Geometry check sheet. Reference: the model listing, model coordinates, mm. A direction names the side the tool comes from. Coordinates: 2 decimals unless noted, no trailing zeros. Loops run counter-clockwise (first coordinate to the right, second up) from the corner with the lowest first, then second, coordinate; pieces in that order, holes last. Notation, with made-up numbers: (-16, 62.25) - (32, 62.25) arc R36 cw to (32, 99.25) - close; hole circle Ø2 at (0, -27.75). An arc over 180 degrees is marked (long way). Write item = value, one per line. Start each with the question number.
from build123d import *

# Parameters (mm, degrees)
F1_W     = 9.495668
F1_H     = 6.474912
F1_W_2   = 9.400923
F1_H_2   = 7.010855
F0_DEPTH = 6.35


with BuildPart() as f0:
    # F1 (on Front) → F0 (new body)
    with BuildSketch(Plane.XZ):
        Polygon((61.962634, 61.060265), (-60.458682, 61.060265), (-60.458682, 55.044476), (44.216055, 55.044476), (44.216055, 22.015698), (61.962634, 22.015698), align=None)
        with Locations((53.525379, 29.250968)):
            Rectangle(F1_W, F1_H, mode=Mode.SUBTRACT)
        with Locations((53.615397, 40.149778)):
            Rectangle(F1_W_2, F1_H_2, mode=Mode.SUBTRACT)
        with Locations((53.615397, 51.539048)):
            Rectangle(F1_W_2, F1_H_2, mode=Mode.SUBTRACT)
    extrude(amount=F0_DEPTH)


solid = f0.part
(1) Depth check by flat-ended pin: pin 1 (1 mm diameter, centred on y = -5, z = 26.5, fed in from -X); pin 2 (3 mm diameter, centred on x = -18.5, y = -4.5, fed in from -Z). Enter the tip coordinate at first touch or a pass-through.
(2) Sectioned sample at B-B on z = 27.5. Enter the section's corners in (x, y).
(3) Sectioned sample at D-D on z = 40.5. Enter the section's corners in (x, y), plus the area to 3 significant figures.
(4) Tool access check on faces 1 (the face through (-9, -3, 55.044)), 2 (the face through (19, -6.35, 58)), 3 (the face through (54, -3, 48.034)). Record the directions out of +Z, -Z, +X, -X, +Y, -Y that give a thin tool (end or side, any length) a straight path to the whole face; none if there is none.
(5) Scan lines: line 1 (X direction, y = -2, z = 26.5); line 2 (X direction, y = -1.5, z = 38.5); line 3 (Z direction, x = 34, y = -4). Record each from-to range of solid material in increasing order.
(6) Sectioned sample at C-C on x = 51. Enter the section's corners in (y, z), plus the area to 3 significant figures.
(7) Sectioned sample at A-A on y = -4. Enter the section's corners in (x, z).
(8) Draft check along X on faces 4 (the face through (53, -3, 32.488)), 5 (the face through (44.216, -3, 39)), 6 (the face through (61.963, -3, 41)). Enter one of: pulls with the +X half, pulls with the -X half, needs draft (parallel to the pull), parting line crosses it, or undercut.
Working result:
q1.pin_1 = 44.22
q1.pin_2 = 55.04
q2.outline = (44.22, -6.35) - (48.78, -6.35) - (48.78, 0) - (44.22, 0) - close; (58.27, -6.35) - (61.96, -6.35) - (61.96, 0) - (58.27, 0) - close
q3.outline = (44.22, -6.35) - (48.91, -6.35) - (48.91, 0) - (44.22, 0) - close; (58.32, -6.35) - (61.96, -6.35) - (61.96, 0) - (58.32, 0) - close
q3.area = 53.0 mm2
q4.face_1 = -Z, -X, +Y, -Y
q4.face_2 = +Z, -Z, +X, -X, -Y
q4.face_3 = +Y, -Y
q5.line_1 = 44.22 to 48.78, 58.27 to 61.96
q5.line_2 = 44.22 to 48.91, 58.32 to 61.96
q5.line_3 = 55.04 to 61.06
q6.outline = (-6.35, 22.02) - (0, 22.02) - (0, 26.01) - (-6.35, 26.01) - close; (-6.35, 32.49) - (0, 32.49) - (0, 36.64) - (-6.35, 36.64) - close; (-6.35, 43.66) - (0, 43.66) - (0, 48.03) - (-6.35, 48.03) - close; (-6.35, 55.04) - (0, 55.04) - (0, 61.06) - (-6.35, 61.06) - close
q6.area = 118 mm2
q7.outline = (-60.46, 55.04) - (44.22, 55.04) - (44.22, 22.02) - (61.96, 22.02) - (61.96, 61.06) - (-60.46, 61.06) - close; hole (48.78, 26.01) - (58.27, 26.01) - (58.27, 32.49) - (48.78, 32.49) - close; hole (48.91, 36.64) - (58.32, 36.64) - (58.32, 43.66) - (48.91, 43.66) - close; hole (48.91, 48.03) - (58.32, 48.03) - (58.32, 55.04) - (48.91, 55.04) - close
q8.face_4 = undercut
q8.face_5 = pulls with the -X half
q8.face_6 = pulls with the +X half
